Source: CAD feature listing. Evaluate the final solid. Frame: model axes, mm. Face numbers are marked on the shaded views. A direction names the side the tool comes from. Coordinates: 2 decimals unless noted, no trailing zeros. Order: outer loops, then holes, each group sorted by start corner. A loop starts at its lowest first (then second) coordinate and runs counter-clockwise, first axis right, second up.
Item 1: Contact query for flat-ended pins moving along their axis: P1, Ø15.5, axis at x = -87, z = 15.5, coming from the +Y side; P2, Ø1.5, axis at x = -13.5, z = 26, coming from the -Y side; P3, Ø12, axis at x = 91, z = 24.5, coming from the +Y side; P4, Ø6, axis at y = 87.5, z = 19.5, coming from the +X side. Output: stop coordinate, or through.
Item 2: Section B-B on y = 48. Return the cut outline in (x, z).
Item 3: Section A-A on x = -29.5. Return the cut outline in (y, z).
Item 4: Mould query, pull axis X, two halves, no side actions, for the marked faces 3, 4 and 5. Classes: released by +X, released by -X, zero draft, split by the parting line, or undercut.
Item 5: Reachability of the marked faces 1 and 2 from +Z, -Z, +X, -X, +Y, -Y: full face, straight path, thin tool, end or side. Return the list, or none.
Item 6: Ray query, line 1 (Y direction, x = 83.5, z = 35.5); line 2 (Y direction, x = 91, z = 32.5); line 3 (X direction, y = -83.5, z = 25.5). Return the intervals inside material, ascending.
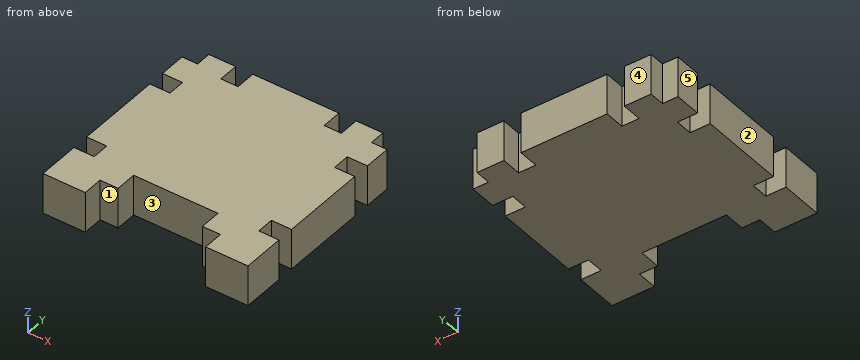
Autodesk Inventor part; units mm, degrees
ref_plane "Plano de trabajo1" through (-100, -100, 39.2) normal (0, 0, 1) x (1, 0, 0)
ref_plane "YZ Plane" through (0, 0, 0) normal (1, 0, 0) x (0, 1, 0)
ref_plane "XZ Plane" through (0, 0, 0) normal (0, 1, 0) x (-1, 0, 0)
sketch "Boceto1" plane through (0, 0, 0) normal (0, 0, 1) x (1, 0, 0)
  line L0 (40.8, -59.2) -> (-40.8, -59.2)
  line L1 (40.8, -79.7) -> (40.8, -59.2)
  line L2 (99.2, -99.2) -> (58.3, -99.2)
  line L3 (99.2, -58.3) -> (99.2, -99.2)
  line L4 (58.3, 99.2) -> (99.2, 99.2)
  line L5 (-99.2, 58.3) -> (-99.2, 99.2)
  line L6 (-58.3, -99.2) -> (-99.2, -99.2)
  line L7 (-40.8, -59.2) -> (-40.8, -79.7)
  line L8 (-40.8, -79.7) -> (-58.3, -79.7)
  line L9 (58.3, -79.7) -> (40.8, -79.7)
  line L10 (58.3, -99.2) -> (58.3, -79.7)
  line L11 (79.7, -58.3) -> (99.2, -58.3)
  line L12 (79.7, -41.7) -> (79.7, -58.3)
  line L13 (99.2, -41.7) -> (79.7, -41.7)
  line L14 (99.2, 41.7) -> (99.2, -41.7)
  line L15 (79.7, 41.7) -> (99.2, 41.7)
  line L16 (79.7, 58.3) -> (79.7, 41.7)
  line L17 (99.2, 58.3) -> (79.7, 58.3)
  line L18 (99.2, 99.2) -> (99.2, 58.3)
  line L19 (58.3, 79.7) -> (58.3, 99.2)
  line L20 (41.7, 79.7) -> (58.3, 79.7)
  line L21 (41.7, 99.2) -> (41.7, 79.7)
  line L22 (-41.7, 99.2) -> (41.7, 99.2)
  line L23 (-41.7, 79.7) -> (-41.7, 99.2)
  line L24 (-58.3, 79.7) -> (-41.7, 79.7)
  line L25 (-58.3, 99.2) -> (-58.3, 79.7)
  line L26 (-99.2, 99.2) -> (-58.3, 99.2)
  line L27 (-79.7, 58.3) -> (-99.2, 58.3)
  line L28 (-79.7, 41.7) -> (-79.7, 58.3)
  line L29 (-99.2, 41.7) -> (-79.7, 41.7)
  line L30 (-99.2, -41.7) -> (-99.2, 41.7)
  line L31 (-79.7, -41.7) -> (-99.2, -41.7)
  line L32 (-79.7, -58.3) -> (-79.7, -41.7)
  line L33 (-99.2, -58.3) -> (-79.7, -58.3)
  line L34 (-99.2, -99.2) -> (-99.2, -58.3)
  line L35 (-58.3, -79.7) -> (-58.3, -99.2)
  line L36 (99.2, 84.2) -> (99.2, 58.3)
  line L37 (84.2, 84.2) -> (99.2, 84.2)
  line L38 (84.2, 99.2) -> (84.2, 84.2)
  line L39 (58.3, 99.2) -> (84.2, 99.2)
  line L40 (58.3, 79.7) -> (58.3, 99.2)
  line L41 (41.7, 79.7) -> (58.3, 79.7)
  line L42 (41.7, 99.2) -> (41.7, 79.7)
  line L43 (-41.7, 99.2) -> (41.7, 99.2)
  line L44 (-41.7, 79.7) -> (-41.7, 99.2)
  line L45 (-58.3, 79.7) -> (-41.7, 79.7)
  line L46 (-58.3, 99.2) -> (-58.3, 79.7)
  line L47 (-84.2, 99.2) -> (-58.3, 99.2)
  line L48 (-84.2, 84.2) -> (-84.2, 99.2)
  line L49 (-99.2, 84.2) -> (-84.2, 84.2)
  line L50 (-99.2, 58.3) -> (-99.2, 84.2)
  line L51 (-79.7, 58.3) -> (-99.2, 58.3)
  line L52 (-79.7, 41.7) -> (-79.7, 58.3)
  line L53 (-99.2, 41.7) -> (-79.7, 41.7)
  line L54 (-99.2, -41.7) -> (-99.2, 41.7)
  line L55 (-79.7, -41.7) -> (-99.2, -41.7)
  line L56 (-79.7, -58.3) -> (-79.7, -41.7)
  line L57 (-99.2, -58.3) -> (-79.7, -58.3)
  line L58 (-99.2, -99.2) -> (-99.2, -58.3)
  line L59 (-58.3, -99.2) -> (-99.2, -99.2)
  line L60 (-58.3, -79.7) -> (-58.3, -99.2)
  line L61 (-40.8, -79.7) -> (-58.3, -79.7)
  line L62 (-40.8, -59.2) -> (-40.8, -79.7)
  line L63 (40.8, -59.2) -> (-40.8, -59.2)
  line L64 (40.8, -79.7) -> (40.8, -59.2)
  line L65 (58.3, -79.7) -> (40.8, -79.7)
  line L66 (58.3, -99.2) -> (58.3, -79.7)
  line L67 (99.2, -99.2) -> (58.3, -99.2)
  line L68 (99.2, -58.3) -> (99.2, -99.2)
  line L69 (79.7, -58.3) -> (99.2, -58.3)
  line L70 (79.7, -41.7) -> (79.7, -58.3)
  line L71 (99.2, -41.7) -> (79.7, -41.7)
  line L72 (99.2, 41.7) -> (99.2, -41.7)
  line L73 (79.7, 41.7) -> (99.2, 41.7)
  line L74 (79.7, 58.3) -> (79.7, 41.7)
  line L75 (99.2, 58.3) -> (79.7, 58.3)
  line L76 (-99.2, 58.3) -> (-99.2, 84.2)
  line L77 (99.2, 84.2) -> (99.2, 58.3)
  line L78 (84.2, 84.2) -> (99.2, 84.2)
  line L79 (84.2, 99.2) -> (84.2, 84.2)
  line L80 (58.3, 99.2) -> (84.2, 99.2)
  line L81 (58.3, 79.7) -> (58.3, 99.2)
  line L82 (41.7, 79.7) -> (58.3, 79.7)
  line L83 (41.7, 99.2) -> (41.7, 79.7)
  line L84 (-41.7, 99.2) -> (41.7, 99.2)
  line L85 (-41.7, 79.7) -> (-41.7, 99.2)
  line L86 (-58.3, 79.7) -> (-41.7, 79.7)
  line L87 (-58.3, 99.2) -> (-58.3, 79.7)
  line L88 (-84.2, 99.2) -> (-58.3, 99.2)
  line L89 (-84.2, 84.2) -> (-84.2, 99.2)
  line L90 (-99.2, 84.2) -> (-84.2, 84.2)
  line L91 (-99.2, 58.3) -> (-99.2, 84.2)
  line L92 (-79.7, 58.3) -> (-99.2, 58.3)
  line L93 (-79.7, 41.7) -> (-79.7, 58.3)
  line L94 (-99.2, 41.7) -> (-79.7, 41.7)
  line L95 (-99.2, -41.7) -> (-99.2, 41.7)
  line L96 (-79.7, -41.7) -> (-99.2, -41.7)
  line L97 (-79.7, -58.3) -> (-79.7, -41.7)
  line L98 (-99.2, -58.3) -> (-79.7, -58.3)
  line L99 (-99.2, -99.2) -> (-99.2, -58.3)
  line L100 (-58.3, -99.2) -> (-99.2, -99.2)
  line L101 (-58.3, -79.7) -> (-58.3, -99.2)
  line L102 (-40.8, -79.7) -> (-58.3, -79.7)
  line L103 (-40.8, -59.2) -> (-40.8, -79.7)
  line L104 (40.8, -59.2) -> (-40.8, -59.2)
  line L105 (40.8, -79.7) -> (40.8, -59.2)
  line L106 (58.3, -79.7) -> (40.8, -79.7)
  line L107 (58.3, -99.2) -> (58.3, -79.7)
  line L108 (99.2, -99.2) -> (58.3, -99.2)
  line L109 (99.2, -58.3) -> (99.2, -99.2)
  line L110 (79.7, -58.3) -> (99.2, -58.3)
  line L111 (79.7, -41.7) -> (79.7, -58.3)
  line L112 (99.2, -41.7) -> (79.7, -41.7)
  line L113 (99.2, 41.7) -> (99.2, -41.7)
  line L114 (79.7, 41.7) -> (99.2, 41.7)
  line L115 (79.7, 58.3) -> (79.7, 41.7)
  line L116 (99.2, 58.3) -> (79.7, 58.3)
  line L117 (99.2, 84.2) -> (99.2, 58.3)
  line L118 (84.2, 84.2) -> (99.2, 84.2)
  line L119 (84.2, 99.2) -> (84.2, 84.2)
  line L120 (58.3, 99.2) -> (84.2, 99.2)
  line L121 (58.3, 79.7) -> (58.3, 99.2)
  line L122 (41.7, 79.7) -> (58.3, 79.7)
  line L123 (41.7, 99.2) -> (41.7, 79.7)
  line L124 (-41.7, 99.2) -> (41.7, 99.2)
  line L125 (-41.7, 79.7) -> (-41.7, 99.2)
  line L126 (-58.3, 79.7) -> (-41.7, 79.7)
  line L127 (-58.3, 99.2) -> (-58.3, 79.7)
  line L128 (-84.2, 99.2) -> (-58.3, 99.2)
  line L129 (-84.2, 84.2) -> (-84.2, 99.2)
  line L130 (-99.2, 84.2) -> (-84.2, 84.2)
  line L131 (-99.2, 58.3) -> (-99.2, 84.2)
  line L132 (-79.7, 58.3) -> (-99.2, 58.3)
  line L133 (-79.7, 41.7) -> (-79.7, 58.3)
  line L134 (-99.2, 41.7) -> (-79.7, 41.7)
  line L135 (-99.2, -41.7) -> (-99.2, 41.7)
  line L136 (-79.7, -41.7) -> (-99.2, -41.7)
  line L137 (-79.7, -58.3) -> (-79.7, -41.7)
  line L138 (-99.2, -58.3) -> (-79.7, -58.3)
  line L139 (-99.2, -99.2) -> (-99.2, -58.3)
  line L140 (-58.3, -99.2) -> (-99.2, -99.2)
  line L141 (-58.3, -79.7) -> (-58.3, -99.2)
  line L142 (-40.8, -79.7) -> (-58.3, -79.7)
  line L143 (-40.8, -59.2) -> (-40.8, -79.7)
  line L144 (40.8, -59.2) -> (-40.8, -59.2)
  line L145 (40.8, -79.7) -> (40.8, -59.2)
  line L146 (58.3, -79.7) -> (40.8, -79.7)
  line L147 (58.3, -99.2) -> (58.3, -79.7)
  line L148 (99.2, -99.2) -> (58.3, -99.2)
  line L149 (99.2, -58.3) -> (99.2, -99.2)
  line L150 (79.7, -58.3) -> (99.2, -58.3)
  line L151 (79.7, -41.7) -> (79.7, -58.3)
  line L152 (99.2, -41.7) -> (79.7, -41.7)
  line L153 (99.2, 41.7) -> (99.2, -41.7)
  line L154 (79.7, 41.7) -> (99.2, 41.7)
  line L155 (79.7, 58.3) -> (79.7, 41.7)
  line L156 (99.2, 58.3) -> (79.7, 58.3)
  point P0 (0, 0)
ref_plane "Plano de trabajo1" through (-100, -100, 39.2) normal (0, 0, 1) x (1, 0, 0)
extrude "Extrusión1" add sketch "Boceto1" along normal up to surface (39.2 mm away) contours L0 L7 L8 L35 L6 L34 L33 L32 L31 L30 L29 L28 L27 L5 L49 L48 L26 L25 L24 L23 L22 L21 L20 L19 L4 L38 L37 L18 L17 L16 L15 L14 L13 L12 L11 L3 L2 L10 L9 L1
properties part number "Cemento"
Answer list:
1. P1: stops at y = 99.2
1. P2: stops at y = -59.2
1. P3: stops at y = 84.2
1. P4: stops at x = 84.2
2. outline: (-79.7, 0) - (79.7, 0) - (79.7, 39.2) - (-79.7, 39.2) - close
3. outline: (-59.2, 0) - (99.2, 0) - (99.2, 39.2) - (-59.2, 39.2) - close
4. face 3: undercut
4. face 4: zero draft
4. face 5: released by -X
5. face 1: +Z, -Z, -Y
5. face 2: +Z, -Z, -X, +Y, -Y
6. line 1: y = -99.2 to -58.3, -41.7 to 41.7, 58.3 to 99.2
6. line 2: y = -99.2 to -58.3, -41.7 to 41.7, 58.3 to 84.2
6. line 3: x = -99.2 to -58.3, 58.3 to 99.2
